Geometry: final body of the model. Coordinates: model frame, mm. Give positions to 0.01 mm unless a question says otherwise; leave off trailing zeros. Order: outer loops, then holes, each group sorted by start corner. A loop starts at its lowest first (then second) coordinate and runs counter-clockwise, first axis right, second up. Notation, with made-up numbers: (-34, 39.25) -> (-20, 39.25) arc R10 cw to (-20, 47.25) -> close; hole circle Ø9 at (-24, -25.75). An arc over 180 degrees is marked (long way). One line per question, with ' | ' between items.
from build123d import *

# Parameters (mm, degrees)
F0_R     = 140
F0_R_2   = 120
F1_DEPTH = 150
F3_DEPTH = 25
F5_DEPTH = 25


with BuildPart() as f1:
    # F0 (on Top) → F1 (new body)
    with BuildSketch(Plane.XY):
        Circle(F0_R)
        Circle(F0_R_2, mode=Mode.SUBTRACT)
    extrude(amount=F1_DEPTH)

    # F2 (on face) → F3 (cut)
    with BuildSketch(Plane.XY.offset(150)):
        with BuildLine():
            ThreePointArc((-91.923882, 91.923882), (-91.035749, 92.803515), (-90.139199, 93.674569))
            ThreePointArc((-90.139199, 93.674569), (-93.691649, 93.691649), (-93.674569, 90.139199))
            ThreePointArc((-93.674569, 90.139199), (-92.803515, 91.035749), (-91.923882, 91.923882))
        make_face()
        with BuildLine():
            Line((-90.156115, 90.156115), (-91.923882, 91.923882))
            ThreePointArc((-91.923882, 91.923882), (-92.803515, 91.035749), (-93.674569, 90.139199))
            ThreePointArc((-93.674569, 90.139199), (-91.911862, 89.42391), (-90.156115, 90.156115))
        make_face()
        with BuildLine():
            ThreePointArc((-89.423882, 91.923882), (-89.60961, 92.869475), (-90.139199, 93.674569))
            ThreePointArc((-90.139199, 93.674569), (-91.035749, 92.803515), (-91.923882, 91.923882))
            Line((-91.923882, 91.923882), (-90.156115, 90.156115))
            ThreePointArc((-90.156115, 90.156115), (-89.614183, 90.967173), (-89.423882, 91.923882))
        make_face()
        with BuildLine():
            ThreePointArc((91.923882, 91.923882), (92.803515, 91.035749), (93.674569, 90.139199))
            ThreePointArc((93.674569, 90.139199), (94.228954, 90.95608), (94.423882, 91.923882))
            ThreePointArc((94.423882, 91.923882), (92.869475, 94.238153), (90.139199, 93.674569))
            ThreePointArc((90.139199, 93.674569), (91.035749, 92.803515), (91.923882, 91.923882))
        make_face()
        with BuildLine():
            Line((90.156115, 90.156115), (91.923882, 91.923882))
            ThreePointArc((91.923882, 91.923882), (91.035749, 92.803515), (90.139199, 93.674569))
            ThreePointArc((90.139199, 93.674569), (89.42391, 91.911862), (90.156115, 90.156115))
        make_face()
        with BuildLine():
            ThreePointArc((90.156115, 90.156115), (91.911862, 89.42391), (93.674569, 90.139199))
            ThreePointArc((93.674569, 90.139199), (92.803515, 91.035749), (91.923882, 91.923882))
            Line((91.923882, 91.923882), (90.156115, 90.156115))
        make_face()
        with BuildLine():
            ThreePointArc((90.139199, -93.674569), (91.035749, -92.803515), (91.923882, -91.923882))
            Line((91.923882, -91.923882), (90.156115, -90.156115))
            ThreePointArc((90.156115, -90.156115), (89.42391, -91.911862), (90.139199, -93.674569))
        make_face()
        with BuildLine():
            ThreePointArc((91.923882, -91.923882), (92.803515, -91.035749), (93.674569, -90.139199))
            ThreePointArc((93.674569, -90.139199), (91.911862, -89.42391), (90.156115, -90.156115))
            Line((90.156115, -90.156115), (91.923882, -91.923882))
        make_face()
        with BuildLine():
            ThreePointArc((94.423882, -91.923882), (94.228954, -90.95608), (93.674569, -90.139199))
            ThreePointArc((93.674569, -90.139199), (92.803515, -91.035749), (91.923882, -91.923882))
            ThreePointArc((91.923882, -91.923882), (91.035749, -92.803515), (90.139199, -93.674569))
            ThreePointArc((90.139199, -93.674569), (92.869475, -94.238153), (94.423882, -91.923882))
        make_face()
        with BuildLine():
            ThreePointArc((-91.923882, -91.923882), (-91.035749, -92.803515), (-90.139199, -93.674569))
            ThreePointArc((-90.139199, -93.674569), (-89.60961, -92.869475), (-89.423882, -91.923882))
            ThreePointArc((-89.423882, -91.923882), (-89.614183, -90.967173), (-90.156115, -90.156115))
            Line((-90.156115, -90.156115), (-91.923882, -91.923882))
        make_face()
        with BuildLine():
            ThreePointArc((-93.674569, -90.139199), (-92.803515, -91.035749), (-91.923882, -91.923882))
            Line((-91.923882, -91.923882), (-90.156115, -90.156115))
            ThreePointArc((-90.156115, -90.156115), (-91.911862, -89.42391), (-93.674569, -90.139199))
        make_face()
        with BuildLine():
            ThreePointArc((-93.674569, -90.139199), (-93.691649, -93.691649), (-90.139199, -93.674569))
            ThreePointArc((-90.139199, -93.674569), (-91.035749, -92.803515), (-91.923882, -91.923882))
            ThreePointArc((-91.923882, -91.923882), (-92.803515, -91.035749), (-93.674569, -90.139199))
        make_face()
    extrude(amount=-F3_DEPTH, mode=Mode.SUBTRACT)

    # F4 (on face) → F5 (cut)
    with BuildSketch(Plane(origin=(0, 0, 0), x_dir=(1, 0, 0), z_dir=(0, 0, -1))):
        with BuildLine():
            ThreePointArc((-91.923882, 91.923882), (-91.035749, 92.803515), (-90.139199, 93.674569))
            ThreePointArc((-90.139199, 93.674569), (-93.691649, 93.691649), (-93.674569, 90.139199))
            ThreePointArc((-93.674569, 90.139199), (-92.803515, 91.035749), (-91.923882, 91.923882))
        make_face()
        with BuildLine():
            Line((-90.156115, 90.156115), (-91.923882, 91.923882))
            ThreePointArc((-91.923882, 91.923882), (-92.803515, 91.035749), (-93.674569, 90.139199))
            ThreePointArc((-93.674569, 90.139199), (-91.911862, 89.42391), (-90.156115, 90.156115))
        make_face()
        with BuildLine():
            ThreePointArc((-89.423882, 91.923882), (-89.60961, 92.869475), (-90.139199, 93.674569))
            ThreePointArc((-90.139199, 93.674569), (-91.035749, 92.803515), (-91.923882, 91.923882))
            Line((-91.923882, 91.923882), (-90.156115, 90.156115))
            ThreePointArc((-90.156115, 90.156115), (-89.614183, 90.967173), (-89.423882, 91.923882))
        make_face()
        with BuildLine():
            ThreePointArc((-93.674569, -90.139199), (-92.803515, -91.035749), (-91.923882, -91.923882))
            Line((-91.923882, -91.923882), (-90.156115, -90.156115))
            ThreePointArc((-90.156115, -90.156115), (-91.911862, -89.42391), (-93.674569, -90.139199))
        make_face()
        with BuildLine():
            ThreePointArc((-91.923882, -91.923882), (-91.035749, -92.803515), (-90.139199, -93.674569))
            ThreePointArc((-90.139199, -93.674569), (-89.60961, -92.869475), (-89.423882, -91.923882))
            ThreePointArc((-89.423882, -91.923882), (-89.614183, -90.967173), (-90.156115, -90.156115))
            Line((-90.156115, -90.156115), (-91.923882, -91.923882))
        make_face()
        with BuildLine():
            ThreePointArc((-93.674569, -90.139199), (-93.691649, -93.691649), (-90.139199, -93.674569))
            ThreePointArc((-90.139199, -93.674569), (-91.035749, -92.803515), (-91.923882, -91.923882))
            ThreePointArc((-91.923882, -91.923882), (-92.803515, -91.035749), (-93.674569, -90.139199))
        make_face()
        with BuildLine():
            ThreePointArc((94.423882, -91.923882), (94.228954, -90.95608), (93.674569, -90.139199))
            ThreePointArc((93.674569, -90.139199), (92.803515, -91.035749), (91.923882, -91.923882))
            ThreePointArc((91.923882, -91.923882), (91.035749, -92.803515), (90.139199, -93.674569))
            ThreePointArc((90.139199, -93.674569), (92.869475, -94.238153), (94.423882, -91.923882))
        make_face()
        with BuildLine():
            ThreePointArc((91.923882, -91.923882), (92.803515, -91.035749), (93.674569, -90.139199))
            ThreePointArc((93.674569, -90.139199), (91.911862, -89.42391), (90.156115, -90.156115))
            Line((90.156115, -90.156115), (91.923882, -91.923882))
        make_face()
        with BuildLine():
            ThreePointArc((90.139199, -93.674569), (91.035749, -92.803515), (91.923882, -91.923882))
            Line((91.923882, -91.923882), (90.156115, -90.156115))
            ThreePointArc((90.156115, -90.156115), (89.42391, -91.911862), (90.139199, -93.674569))
        make_face()
        with BuildLine():
            Line((90.156115, 90.156115), (91.923882, 91.923882))
            ThreePointArc((91.923882, 91.923882), (91.035749, 92.803515), (90.139199, 93.674569))
            ThreePointArc((90.139199, 93.674569), (89.42391, 91.911862), (90.156115, 90.156115))
        make_face()
        with BuildLine():
            ThreePointArc((90.156115, 90.156115), (91.911862, 89.42391), (93.674569, 90.139199))
            ThreePointArc((93.674569, 90.139199), (92.803515, 91.035749), (91.923882, 91.923882))
            Line((91.923882, 91.923882), (90.156115, 90.156115))
        make_face()
        with BuildLine():
            ThreePointArc((91.923882, 91.923882), (92.803515, 91.035749), (93.674569, 90.139199))
            ThreePointArc((93.674569, 90.139199), (94.228954, 90.95608), (94.423882, 91.923882))
            ThreePointArc((94.423882, 91.923882), (92.869475, 94.238153), (90.139199, 93.674569))
            ThreePointArc((90.139199, 93.674569), (91.035749, 92.803515), (91.923882, 91.923882))
        make_face()
    extrude(amount=-F5_DEPTH, mode=Mode.SUBTRACT)


solid = f1.part
1) Section A-A on x = 0. Return loops of the section in (y, z), plus the area to 3 significant figures.
Check result:
outline: (-140, 0) -> (-120, 0) -> (-120, 150) -> (-140, 150) -> close; (120, 0) -> (140, 0) -> (140, 150) -> (120, 150) -> close | area: 6,000 mm^2
2) Material intervals for probe 1 along Y at (x, z) = (0, 46); probe 2 along Y at (x, z) = (90, 11), sorted ascending. Write a range as from..to.
Check result:
probe 1: y = -140..-120, 120..140 | probe 2: y = -107.24..-93.52, -90.33..-79.37, 79.37..90.33, 93.52..107.24
3) Section D-D on z = 54. Return loops of the section in (x, y), plus the area to 3 significant figures.
Check result:
outline: circle Ø280 at (0, 0); hole circle Ø240 at (0, 0) | area: 16,300 mm^2
4) Pull-direction query (X, two-part tool) for faces 1 (the cylindrical face through (-111.1, -85.19, 73.95)), 2 (the flat face through (103, -62, 150)), 3 (the cylindrical face through (-119.884, 5.276, 73.95)); classes: +X half, -X half, draft (parallel to the pull), parting line (faces both ways), or undercut.
Check result:
face 1: parting line | face 2: draft | face 3: undercut
5) Section C-C on z = 14. Return loops of the section in (x, y), plus the area to 3 significant figures.
Check result:
outline: circle Ø280 at (0, 0); hole circle Ø240 at (0, 0); hole (-93.67, -90.14) arc R2.5 ccw (long way) to (-90.14, -93.67) arc R2.5 ccw to (-89.42, -91.92) arc R2.5 ccw to (-90.16, -90.16) arc R2.5 ccw to start; hole (-93.67, 90.14) arc R2.5 ccw to (-90.16, 90.16) arc R2.5 ccw to (-89.42, 91.92) arc R2.5 ccw to (-90.14, 93.67) arc R2.5 ccw (long way) to start; hole (90.14, -93.67) arc R2.5 ccw to (94.42, -91.92) arc R2.5 ccw to (93.67, -90.14) arc R2.5 ccw to (90.16, -90.16) arc R2.5 ccw to start; hole (90.14, 93.67) arc R2.5 ccw to (90.16, 90.16) arc R2.5 ccw to (93.67, 90.14) arc R2.5 ccw to (94.42, 91.92) arc R2.5 ccw to start | area: 16,300 mm^2
6) Contact query for flat-ended pins moving along their axis: pin 1 Ø10 at (x, z) = (16.5, 84) entering from +Y; pin 2 Ø12 at (y, z) = (91, 91) entering from -X; pin 3 Ø1.5 at (x, y) = (-92.5, 91.5) entering from -Z. Output: stop coordinate, or through.
Check result:
pin 1: stops at y = 139.53 | pin 2: stops at x = -111.24 | pin 3: stops at z = 25
